from build123d import *

# Parameters (mm, degrees)
SKETCH1_R               = 2
BOSS_EXTRUDE1_DEPTH     = 20
SKETCH2_R               = 1.5
CUT_EXTRUDE1_DEPTH      = 3
CUT_EXTRUDE1_DEPTH_BACK = 3
FILLET1_R               = 0.5


with BuildPart() as part:
    # Sketch1 → Boss-Extrude1 (new body)
    with BuildSketch(Plane.XY):
        Circle(SKETCH1_R)
    extrude(amount=BOSS_EXTRUDE1_DEPTH)

    # Sketch2 → Cut-Extrude1 (cut, two sides)
    with BuildSketch(Plane(origin=(0, 0, 0), x_dir=(1, 0, 0), z_dir=(0, 1, 0))) as cut_extrude1_sk:
        with Locations((0, -17.5)):
            Circle(SKETCH2_R)
    extrude(amount=CUT_EXTRUDE1_DEPTH, mode=Mode.SUBTRACT)
    extrude(cut_extrude1_sk.sketch, amount=-CUT_EXTRUDE1_DEPTH_BACK, mode=Mode.SUBTRACT)

    # Fillet1
    fillet1_edges = [part.edges().sort_by_distance(p)[0] for p in [
        (-2, 0, 0),
        (-2, 0, 20),
    ]]
    fillet(fillet1_edges, radius=FILLET1_R)


solid = part.part
CAD build for the part. Positions are in the model's coordinates, mm. Give positions to 0.01 mm unless a question says otherwise; leave off trailing zeros. Loops run counter-clockwise (first coordinate to the right, second up) from the corner with the lowest first, then second, coordinate; pieces in that order, holes last. Notation, with made-up numbers: M -17,75 L -9,75 A7 cw -9,84 Z; hole C 23,38 d3. An arc over 180 degrees is marked long. One line per question, with ' | ' between items. Start each with the question number.
1. Probe L1, parallel to Z at x = 0, y = 0.9; L2, parallel to Z at x = -0.8, y = 0.3; L3, parallel to X at y = -0.45, z = 17.5. List the from-to ranges inside material, lowest first. Write a range as from..to.
2. Flat gauge pin, fed straight in: pin 1 (1 mm diameter, centred on y = 1, z = 5.5, fed in from +X). Where does the tip first touch, or does it go through?
3. Saw through at A-A on x = 0. Give the cut face in (y, z), plus the area to 3 significant figures.
4. Saw through at C-C on z = 9. Give the cut face in (x, y).
5. Saw through at B-B on z = 17.5. Give the cut face in (x, y), plus the area to 3 significant figures.
Result sheet:
1) L1: z = 0..16, 19..20 | L2: z = 0..16.23, 18.77..20 | L3: x = -1.95..-1.5, 1.5..1.95
2) pin 1: stops at x = 1.94
3) outline: M -2,0.5 A0.5 ccw -1.5,0 L 1.5,0 A0.5 ccw 2,0.5 L 2,16 L -2,16 Z; M -2,19 L 2,19 L 2,19.5 A0.5 ccw 1.5,20 L -1.5,20 A0.5 ccw -2,19.5 Z | area: 67.8 mm^2
4) outline: C 0,0 d4
5) outline: M -1.5,-1.32 L -1.5,1.32 A2 ccw Z; M 1.5,-1.32 A2 ccw 1.5,1.32 Z | area: 1.81 mm^2
